Verification items for the finished model (mm, model axes). Face numbers are marked on the shaded views. Coordinates: 2 decimals unless noted, no trailing zeros. Write each loop counter-clockwise with the first axis right and the second up, starting at its lowest first coordinate (ties: lowest second). Pieces come first, ordered by that corner, then holes. Notation, with made-up numbers: (-34, 83.5) -> (-6, 83.5) arc R11 ccw to (-6, 97.5) -> close; hole circle Ø5 at (-8.75, 31). An arc over 180 degrees is marked (long way). Use a Markdown table: item, result. Add a question column.
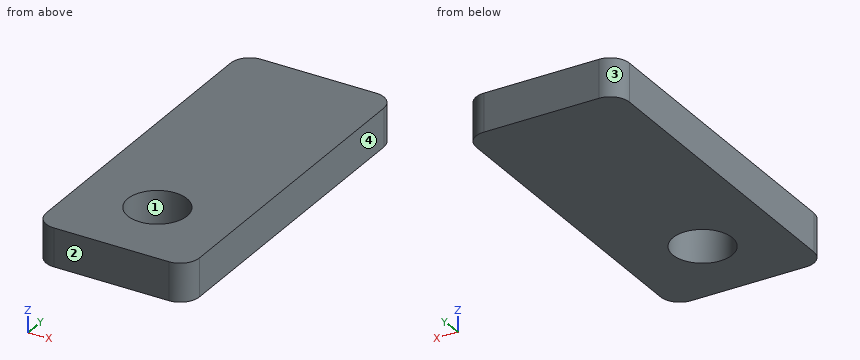
from build123d import *

# Parameters (mm, degrees)
SKETCH_1_R      = 1.55
EXTRUDE_1_DEPTH = 2


with BuildPart() as part:
    # 草图1 → 凸台-拉伸1 (new body)
    with BuildSketch(Plane.XY):
        with BuildLine():
            Line((-3, 9), (3, 9))
            ThreePointArc((3, 9), (3.707106781, 8.707106781), (4, 8))
            Line((4, 8), (4, -8))
            ThreePointArc((4, -8), (3.707106781, -8.707106781), (3, -9))
            Line((3, -9), (-3, -9))
            ThreePointArc((-3, -9), (-3.707106781, -8.707106781), (-4, -8))
            Line((-4, -8), (-4, 8))
            ThreePointArc((-4, 8), (-3.707106781, 8.707106781), (-3, 9))
        make_face()
        with Locations((0, -5)):
            Circle(SKETCH_1_R, mode=Mode.SUBTRACT)
    extrude(amount=EXTRUDE_1_DEPTH)


solid = part.part
1) Gauge pin test, flat end, axial feed: pin 1 (1.5 mm diameter, centred on x = -3, y = 4.5, fed in from -Z). Record the tip position at first contact, or that the pin passes through.
2) Cross-section at C-C on z = 1.3. Record the boundary of the cut face in (x, y).
3) Thickness scan on L1, parallel to Y at x = 0, z = 0.5; L2, parallel to X at y = -4, z = 1.75; L3, parallel to Y at x = 0.75, z = 1.45. Record the ranges inside material, lowest first.
4) Cross-section at A-A on x = 0. Record the boundary of the cut face in (y, z).
5) Cross-section at B-B on y = -5. Record the boundary of the cut face in (x, z), then the cut area to 3 significant figures.
6) Release check for a two-part mould opening along Y. For the marked faces 1, 2, 3 and 4 record: released by +Y, released by -Y, zero draft, split by the parting line, or undercut.
Returned:
| question | item | result |
|---|---|---|
| 1 | pin 1 | stops at z = 0 |
| 2 | outline | (-4, -8) arc R1 ccw to (-3, -9) -> (3, -9) arc R1 ccw to (4, -8) -> (4, 8) arc R1 ccw to (3, 9) -> (-3, 9) arc R1 ccw to (-4, 8) -> close; hole circle Ø3.1 at (0, -5) |
| 3 | L1 | y = -9 to -6.55, -3.45 to 9 |
| 3 | L2 | x = -4 to -1.18, 1.18 to 4 |
| 3 | L3 | y = -9 to -6.36, -3.64 to 9 |
| 4 | outline | (-9, 0) -> (-6.55, 0) -> (-6.55, 2) -> (-9, 2) -> close; (-3.45, 0) -> (9, 0) -> (9, 2) -> (-3.45, 2) -> close |
| 5 | outline | (-4, 0) -> (-1.55, 0) -> (-1.55, 2) -> (-4, 2) -> close; (1.55, 0) -> (4, 0) -> (4, 2) -> (1.55, 2) -> close |
| 5 | area | 9.80 mm² |
| 6 | face 1 | undercut |
| 6 | face 2 | released by -Y |
| 6 | face 3 | released by +Y |
| 6 | face 4 | zero draft |
